The model under review builds one solid part; all positions refer to its coordinate system, in mm. A direction names the side the tool comes from. Round coordinates to 2 decimals unless told otherwise and drop trailing zeros. Order: outer loops, then holes, each group sorted by start corner. A loop starts at its lowest first (then second) coordinate and runs counter-clockwise, first axis right, second up.
1) Machinability: for faces 4 (the face through (-13, -46.99, -4)), 5 (the face through (-13, -68, -5.461)), 6 (the face through (10.16, -68, -4)), which of the approach directions +Z, -Z, +X, -X, +Y, -Y give a long, thin tool a straight path to every point of the face, cutting with its end or side? Answer none if there is none.
2) Consider section B-B (y = -24.5). Give the boundary of the cut face in (x, z) (3 decimals).
3) To check wall thickness, follow L1, parallel to Z at x = 0, y = -59; L2, parallel to Y at x = 14, z = -3; L3, parallel to Z at x = 1, y = -59. State the ranges of each line that lie inside material, in increasing order.
4) Clearance check with flat-ended pins moving along their axes: P1, Ø8, axis at x = -2, y = -25.5, coming from the -Z side; P2, Ø0.8, axis at x = -13, y = -46, coming from the -Z side. State where each tip first meets the part, or that it passes through.
5) Consider section C-C (z = 3.5). Give the boundary of the cut face in (x, y).
6) Consider section D-D (x = 13). Give the boundary of the cut face in (y, z).
7) Mouldability with a two-part tool opening along X and no side actions: class faces 1 (the face through (-13, -44.45, -4)), 2 (the face through (0, -44, 0)), 3 (the face through (13.712, -45.072, 4.901)) as pulls with the +X half, pulls with the -X half, needs draft (parallel to the pull), parting line crosses it, or undercut.
8) Consider section A-A (x = 0). Give the boundary of the cut face in (y, z), then the cut area to 3 significant figures.
from build123d import *

# Parameters (mm, degrees)
F0_R          = 2.286
F1_DEPTH      = 88.9
F2_R          = 1.27
F3_R          = 5.08
F4_W          = 2.54
F4_H          = 3.0299487758
F5_DEPTH      = 5.081
F5_DEPTH_BACK = 25.401


with BuildPart() as f1:
    # F0 (on Front) → F1 (new body)
    with BuildSketch(Plane.XZ):
        Polygon((-12.065, 0), (0, 0), (12.065, 0), (10.16, -1.905), (10.16, -5.461), (15.24, -5.461), (15.24, 6.35), (0, 6.35), (-15.24, 6.35), (-15.24, -5.461), (-10.16, -5.461), (-10.16, -1.905), align=None)
        with Locations((0, 2.54)):
            Circle(F0_R, mode=Mode.SUBTRACT)
    extrude(amount=F1_DEPTH)

    # F2
    f2_edges = [f1.edges().sort_by_distance(p)[0] for p in [
        (-10.16, -44.45, -1.905),
        (10.16, -44.45, -1.905),
    ]]
    fillet(f2_edges, radius=F2_R)

    # F3
    f3_edges = [f1.edges().sort_by_distance(p)[0] for p in [
        (-15.24, -44.45, 6.35),
        (15.24, -44.45, 6.35),
    ]]
    fillet(f3_edges, radius=F3_R)

    # F4 (on face) → F5 (cut, two sides)
    with BuildSketch(Plane.YZ.offset(-10.16)) as f5_sk:
        with Locations((-45.72, -3.9460256121)):
            Rectangle(F4_W, F4_H)
    extrude(amount=-F5_DEPTH, mode=Mode.SUBTRACT)
    extrude(f5_sk.sketch, amount=F5_DEPTH_BACK, mode=Mode.SUBTRACT)


solid = f1.part
Answer below:
1. face 4: -Z, +X, -X
1. face 5: -Z, +X, -X, +Y, -Y
1. face 6: -Z, +Y, -Y
2. outline: (-15.24, -5.461) - (-10.16, -5.461) - (-10.16, -2.431) arc R1.27 ccw to (-10.532, -1.533) - (-12.065, 0) - (12.065, 0) - (10.532, -1.533) arc R1.27 ccw to (10.16, -2.431) - (10.16, -5.461) - (15.24, -5.461) - (15.24, 1.27) arc R5.08 ccw to (10.16, 6.35) - (-10.16, 6.35) arc R5.08 ccw to (-15.24, 1.27) - close; hole circle Ø4.572 at (0, 2.54)
3. L1: z = 0 to 0.25, 4.83 to 6.35
3. L2: y = -88.9 to -46.99, -44.45 to 0
3. L3: z = 0 to 0.48, 4.6 to 6.35
4. P1: stops at z = 0
4. P2: stops at z = -2.43
5. outline: (-14.72, -88.9) - (-2.07, -88.9) - (-2.07, 0) - (-14.72, 0) - close; (2.07, -88.9) - (14.72, -88.9) - (14.72, 0) - (2.07, 0) - close
6. outline: (-88.9, -5.46) - (-46.99, -5.46) - (-46.99, -2.43) - (-44.45, -2.43) - (-44.45, -5.46) - (0, -5.46) - (0, 5.48) - (-88.9, 5.48) - close
7. face 1: needs draft
7. face 2: undercut
7. face 3: pulls with the +X half
8. outline: (-88.9, 0) - (0, 0) - (0, 0.25) - (-88.9, 0.25) - close; (-88.9, 4.83) - (0, 4.83) - (0, 6.35) - (-88.9, 6.35) - close
8. area: 158 mm2
